Geometry: see drawing. Coordinates: mm, zero at the bounding-box minimum. Coordinates: 2 decimals unless noted, no trailing zeros. Order: outer loops, then holes, each group sorted by start corner. A loop starts at its lowest first (then second) coordinate and runs counter-clockwise, first axis right, second up. Notation, with made-up numbers: (79.25, -5.5) -> (98.25, -5.5) arc R26 ccw to (98.25, 21.5) -> close; hole circle Ø7 at (-39, -6). An arc over 180 degrees is marked (long way). Use one line per item in the form item = value.
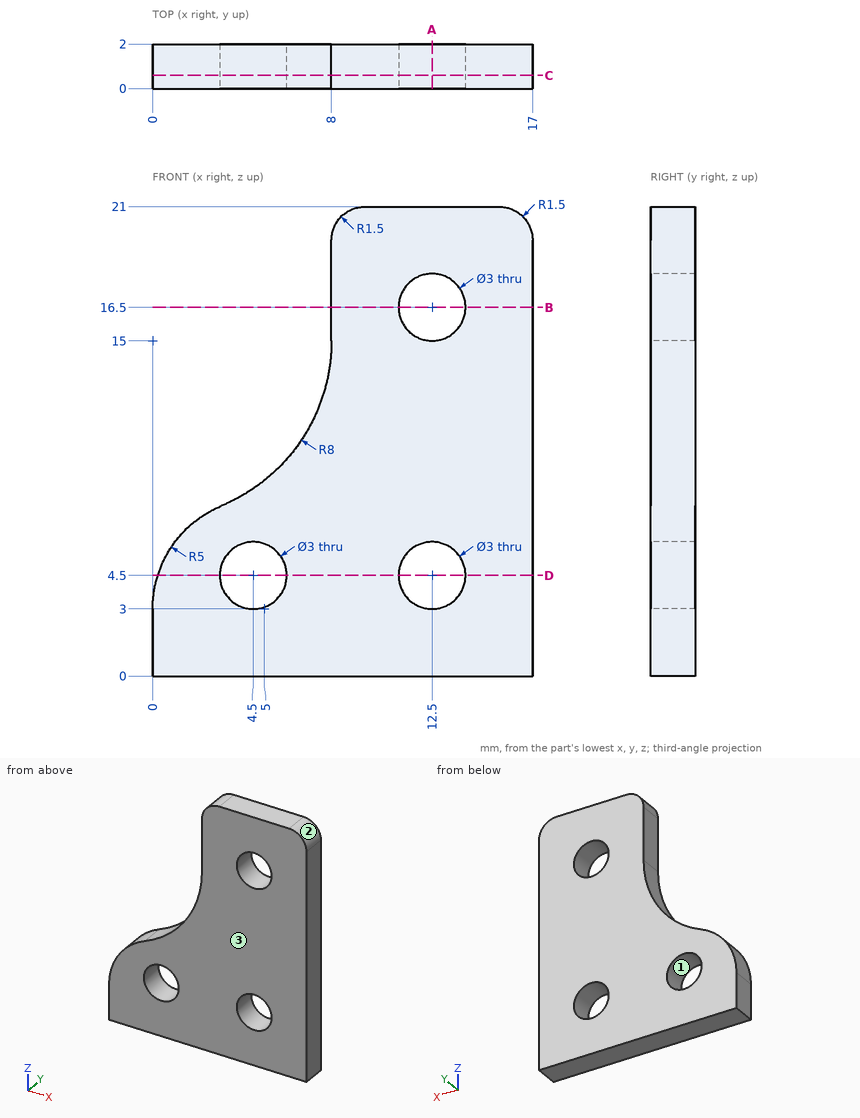
1) Section C-C, the plane y = 0.6. Output: boundary loops of the cut face in (x, z).
Results found:
outline = (0, 0) -> (17, 0) -> (17, 19.5) arc R1.5 ccw to (15.5, 21) -> (9.5, 21) arc R1.5 ccw to (8, 19.5) -> (8, 15) arc R8 cw to (3.08, 7.62) arc R5 ccw to (0, 3) -> close; hole circle Ø3 at (4.5, 4.5); hole circle Ø3 at (12.5, 4.5); hole circle Ø3 at (12.5, 16.5)
2) Section D-D, the plane z = 4.5. Output: boundary loops of the cut face in (x, y).
Results found:
outline = (0.23, 0) -> (3, 0) -> (3, 2) -> (0.23, 2) -> close; (6, 0) -> (11, 0) -> (11, 2) -> (6, 2) -> close; (14, 0) -> (17, 0) -> (17, 2) -> (14, 2) -> close
3) Material intervals for probe 1 along Z at (x, y) = (12.5, 0.9); probe 2 along X at (y, z) = (1.9, 4.25); probe 3 along Z at (x, y) = (4.5, 1.45), sorted ascending. Write a range as from..to.
Results found:
probe_1 = 0..3, 6..15, 18..21
probe_2 = 0.16..3.02, 5.98..11.02, 13.98..17
probe_3 = 0..3, 6..8.39
4) Section A-A, the plane x = 12.5. Output: boundary loops of the cut face in (y, z), and give its area (3 significant figures).
Results found:
outline = (0, 0) -> (2, 0) -> (2, 3) -> (0, 3) -> close; (0, 6) -> (2, 6) -> (2, 15) -> (0, 15) -> close; (0, 18) -> (2, 18) -> (2, 21) -> (0, 21) -> close
area = 30.0 mm2
5) Pull-direction query (Z, two-part tool) for the marked faces 1, 2 and 3; classes: released by +Z, released by -Z, zero draft, split by the parting line, or undercut.
Results found:
face_1 = undercut
face_2 = released by +Z
face_3 = zero draft
6) Section B-B, the plane z = 16.5. Output: boundary loops of the cut face in (x, y), and give its area (3 significant figures).
Results found:
outline = (8, 0) -> (11, 0) -> (11, 2) -> (8, 2) -> close; (14, 0) -> (17, 0) -> (17, 2) -> (14, 2) -> close
area = 12.0 mm2
